Design review of the part built by this model. Coordinates are the model's own, in mm. Give positions to 0.01 mm unless a question says otherwise; leave off trailing zeros. Write each loop counter-clockwise with the first axis right and the second up, starting at its lowest first coordinate (ties: lowest second). Pieces come first, ordered by that corner, then holes. Notation, with made-up numbers: (76, -17.5) -> (133, -17.5) arc R9 ccw to (133, -3.5) -> close; hole circle Ø9 at (35.5, 29). An arc over 180 degrees is marked (long way). Put each result on its own line as item: value. Start each with the question number.
Autodesk Inventor part; units mm, degrees
ref_plane "YZ Plane" through (0, 0, 0) normal (1, 0, 0) x (0, 1, 0)
ref_plane "XZ Plane" through (0, 0, 0) normal (0, 1, 0) x (-1, 0, 0)
ref_plane "XY Plane" through (0, 0, 0) normal (0, 0, 1) x (1, 0, 0)
sketch "Sketch1" plane through (0, 0, 0) normal (0, 0, 1) x (1, 0, 0)
  circle A0 centre (46.9462, 34.742) radius 1.05
  circle A1 centre (53.415, 34.1058) radius 1.05
  circle A2 centre (-46.9442, -34.742) radius 1.05 construction
  circle A3 centre (-53.413, -34.1058) radius 1.05 construction
  arc A4 (72.8682, -20.1426) -> (68.7671, -31.41) centre (71.0414, -25.8577) ccw
  arc A5 (72.8682, -20.1426) -> (72.8688, 20.1405) centre (0.001, 0) ccw
  arc A6 (68.768, 31.408) -> (72.8688, 20.1405) centre (71.0421, 25.8557) ccw
  arc A7 (68.768, 31.408) -> (61.5859, 43.8482) centre (0.001, 0) ccw
  arc A8 (53.8786, 53.0336) -> (61.5859, 43.8482) centre (57.9147, 48.5939) ccw
  arc A9 (53.8786, 53.0336) -> (42.8749, 62.2671) centre (0.001, 0) ccw
  arc A10 (32.4909, 68.2625) -> (42.8749, 62.2671) centre (37.8019, 65.471) ccw
  arc A11 (32.4909, 68.2625) -> (18.9927, 73.1756) centre (0.001, 0) ccw
  arc A12 (7.1843, 75.258) -> (18.9927, 73.1756) centre (13.1299, 74.4513) ccw
  arc A13 (7.1843, 75.258) -> (-7.1802, 75.2582) centre (0.001, 0) ccw
  arc A14 (-18.9886, 73.1762) -> (-7.1802, 75.2582) centre (-13.1257, 74.4517) ccw
  arc A15 (-18.9886, 73.1762) -> (-32.4869, 68.2634) centre (0.001, 0) ccw
  arc A16 (-42.8711, 62.2683) -> (-32.4869, 68.2634) centre (-37.7981, 65.4721) ccw
  arc A17 (-42.8711, 62.2683) -> (-53.8751, 53.0351) centre (0.001, 0) ccw
  arc A18 (-61.5826, 43.8499) -> (-53.8751, 53.0351) centre (-57.9113, 48.5956) ccw
  arc A19 (-61.5826, 43.8499) -> (-68.7651, 31.41) centre (0.001, 0) ccw
  arc A20 (-72.8662, 20.1426) -> (-68.7651, 31.41) centre (-71.0394, 25.8577) ccw
  arc A21 (-72.8662, 20.1426) -> (-72.8668, -20.1405) centre (0.001, 0) ccw
  arc A22 (-68.766, -31.408) -> (-72.8668, -20.1405) centre (-71.0401, -25.8557) ccw
  arc A23 (-68.766, -31.408) -> (-61.5839, -43.8482) centre (0.001, 0) ccw
  arc A24 (-53.8766, -53.0336) -> (-61.5839, -43.8482) centre (-57.9127, -48.5939) ccw
  arc A25 (-53.8766, -53.0336) -> (-42.8729, -62.2671) centre (0.001, 0) ccw
  arc A26 (-32.4889, -68.2625) -> (-42.8729, -62.2671) centre (-37.7999, -65.471) ccw
  arc A27 (-32.4889, -68.2625) -> (-18.9907, -73.1756) centre (0.001, 0) ccw
  arc A28 (-7.1823, -75.258) -> (-18.9907, -73.1756) centre (-13.1279, -74.4513) ccw
  arc A29 (-7.1823, -75.258) -> (7.1822, -75.2582) centre (0.001, 0) ccw
  arc A30 (18.9906, -73.1762) -> (7.1822, -75.2582) centre (13.1277, -74.4517) ccw
  arc A31 (18.9906, -73.1762) -> (32.4889, -68.2634) centre (0.001, 0) ccw
  arc A32 (42.8731, -62.2683) -> (32.4889, -68.2634) centre (37.8001, -65.4721) ccw
  arc A33 (42.8731, -62.2683) -> (53.8771, -53.0351) centre (0.001, 0) ccw
  arc A34 (61.5846, -43.8499) -> (53.8771, -53.0351) centre (57.9133, -48.5956) ccw
  arc A35 (61.5846, -43.8499) -> (68.7671, -31.41) centre (0.001, 0) ccw
  circle A36 centre (0.001, 0) radius 44.3
  circle A37 centre (-69.9492, -11.499) radius 1.3
  circle A38 centre (-46.9488, 11.5007) radius 1.3
  circle A39 centre (69.9508, -11.501) radius 1.3
  circle A40 centre (46.9512, 11.4993) radius 1.3
  circle A41 centre (69.9512, 11.499) radius 1.3
  circle A42 centre (46.9508, -11.5007) radius 1.3
  circle A43 centre (-69.9488, 11.501) radius 1.3
  circle A44 centre (-46.9492, -11.4993) radius 1.3
  circle A45 centre (-58.449, 0.0008) radius 11.5
  circle A46 centre (58.451, -0.0008) radius 11.5
  circle A47 centre (60.2759, -34.8009) radius 1.55
  circle A48 centre (44.7383, -53.3173) radius 1.55
  circle A49 centre (16.1779, -44.4477) radius 1.55
  circle A50 centre (0, -69.6) radius 1.55
  circle A51 centre (-23.8045, -65.4023) radius 1.55
  circle A52 centre (-30.4034, -36.2335) radius 1.55
  circle A53 centre (-60.2749, -34.7991) radius 1.55
  circle A54 centre (60.2769, 34.7991) radius 1.55
  circle A55 centre (44.7398, 53.3161) radius 1.55
  circle A56 centre (23.8065, 65.4023) radius 1.55
  circle A57 centre (-40.9617, 23.6506) radius 1.55
  circle A58 centre (-30.4023, 36.2343) radius 1.55
  circle A59 centre (-16.1759, 44.4477) radius 1.55
  circle A60 centre (0.0017, 47.3) radius 1.55
  circle A61 centre (0.002, 69.6) radius 1.55
  circle A62 centre (-23.8027, 65.4029) radius 1.55
  circle A63 centre (-44.7363, 53.3173) radius 1.55
  circle A64 centre (-60.2739, 34.8009) radius 1.55
  circle A65 centre (16.1792, 44.4472) radius 1.55
  circle A66 centre (30.4054, 36.2335) radius 1.55
  circle A67 centre (40.9643, 23.6494) radius 1.55
  circle A68 centre (-40.9623, -23.6494) radius 1.55
  circle A69 centre (-44.7378, -53.3161) radius 1.55
  circle A70 centre (-16.1772, -44.4472) radius 1.55
  circle A71 centre (0.0003, -47.3) radius 1.55
  circle A72 centre (23.8047, -65.4029) radius 1.55
  circle A73 centre (30.4043, -36.2343) radius 1.55
  circle A74 centre (40.9637, -23.6506) radius 1.55
  line L0 (58.451, 0) -> (0.001, 0) construction
  line L1 (71.0414, -19.8577) -> (39.601, -19.8577)
  line L2 (0.001, 0) -> (0.001, -87.4041) construction
  line L3 (71.0414, -25.8577) -> (71.0414, -19.8577) construction
  line L4 (39.601, -19.8577) -> (-39.599, -19.8577) construction
  line L5 (-39.599, -19.8577) -> (-71.0397, -19.8557)
  point P0 (0, 0)
extrude "Extrusion1" add sketch "Sketch1" along normal blind 1.75 contours A4 A35 A34 A33 A32 A31 A30 A29 A28 A27 A26 A25 A24 A23 A22 L5 A36 L1
sketch "Sketch2" plane through (0, 0, 1.75) normal (0, 0, 1) x (1, 0, 0)
  circle A0 centre (-30.4034, -36.2335) radius 1.55
  circle A1 centre (-44.7378, -53.3161) radius 1.55
  circle A2 centre (-23.8045, -65.4023) radius 1.55
  circle A3 centre (-16.1772, -44.4472) radius 1.55
  circle A4 centre (16.1779, -44.4477) radius 1.55
  circle A5 centre (23.8047, -65.4029) radius 1.55
  circle A6 centre (44.7383, -53.3173) radius 1.55
  circle A7 centre (30.4043, -36.2343) radius 1.55
  circle A8 centre (0.0003, -47.3) radius 1.55
  point P0 (0, 0)
extrude "Extrusion2" add sketch "Sketch2" against normal up to surface (1.75 mm away)
sketch "Sketch3" plane through (0, 0, 1.75) normal (0, 0, 1) x (1, 0, 0)
  line L0 (-60.9088, -23.5183) -> (-47.1121, -23.5183) construction
  line L1 (-60.9088, -25.0183) -> (-47.1121, -25.0183)
  line L2 (-47.1121, -22.0183) -> (-60.9088, -22.0183)
  arc A0 (-60.9088, -22.0183) -> (-60.9088, -25.0183) centre (-60.9088, -23.5183) ccw
  arc A1 (-47.1121, -25.0183) -> (-47.1121, -22.0183) centre (-47.1121, -23.5183) ccw
  line L3 (-60.9088, -23.5183) -> (-65.5141, -23.5183) construction
  arc A2 (-68.766, -31.408) -> (-71.0397, -19.8557) centre (-71.0401, -25.8557) ccw
  line L4 (-47.1121, -23.5183) -> (-42.5068, -23.5183) construction
  circle A3 centre (-40.9623, -23.6494) radius 1.55
  point P0 (0, 0)
  point P1 (-54.0105, -23.5183)
  point P2 (-71.0401, -19.8557)
  dimension "d4" = 3
extrude "Extrusion3" cut sketch "Sketch3" against normal up to surface (1.75 mm away) contours A0 L2 A1 L1
mirror "Mirror1" about plane through (0, 0, 0) normal (1, 0, 0) of "Extrusion3"
sketch "Sketch4" plane through (0, 0, 1.75) normal (0, 0, 1) x (1, 0, 0)
  line L0 (13.6094, 45.369) -> (8.7511, 46.5508) construction
  line L1 (13.8458, 46.3407) -> (8.9875, 47.5225)
  line L2 (8.5148, 45.5792) -> (13.3731, 44.3973)
  arc A0 (13.3731, 44.3973) -> (13.8458, 46.3407) centre (13.6094, 45.369) ccw
  arc A1 (8.9875, 47.5225) -> (8.5148, 45.5792) centre (8.7511, 46.5508) ccw
  circle A2 centre (0, 0) radius 47.3002 construction
  arc A3 (-39.599, -19.8577) -> (39.601, -19.8577) centre (0.001, 0) ccw
  point P0 (11.1803, 45.9599)
  point P1 (-39.6, -19.8557)
  dimension "d7" = 2
  dimension "d8" = 5
  dimension "d9" = 2
extrude "Extrusion4" cut sketch "Sketch4" against normal up to surface (1.75 mm away)
equation "\"d0\" = board_height"
equation "\"d2\" = board_height"
equation "\"d5\" = board_height"
equation "\"d10\" = board_height"
equation "\"board_height\" = 1.75"
properties part number "Board_Shape"
Q1. Mouldability with a two-part tool opening along Y and no side actions: class faces 1 (the face through (-42.51, -23.72, 0.86)), 2 (the face through (-1, -47, 0)), 3 (the face through (65.522, -37.714, 0.863)) as +Y half, -Y half, draft (parallel to the pull), parting line (faces both ways), or undercut.
Q2. To check wall thickness, follow probe 1 along X at (y, z) = (-35, 0.4); probe 2 along Y at (x, z) = (0, 0.6); probe 3 along X at (y, z) = (-31, 1.7). State the ranges of each line that lie inside material, in increasing order. Write a range as from..to.
Q3. Take a section at B-B on z = 1.05. State how many separate pieces and enclosed holes the cut face has, then the cut area to 3 significant figures.
Q4. Take a section at D-D on x = -16. Give the boundary of the cut face in (y, z), then the cut area to 3 significant figures.
Q5. For pin 1 (1 mm diameter, centred on x = 22, z = 1, fed in from +Y); pin 2 (3.5 mm diameter, centred on x = 0, y = -69.6, fed in from +Z); pin 3 (0.9 mm diameter, centred on x = -53, z = 0.5, fed in from -Y); pin 4 (1 mm diameter, centred on x = 3, z = 1.5, fed in from +Y), all flat-tipped, find the tip position at first contact; note any pin that passes through.
Q6. Take a section at A-A on x = 0. Give the boundary of the cut face in (y, z), then the cut area to 4 significant figures.
Q7. Take a section at C-C on y = -56. Give the boundary of the cut face in (x, z), then the cut area to 3 significant figures.
Result:
1. face 1: undercut
1. face 2: draft
1. face 3: -Y half
2. probe 1: x = -67.01..-61.81, -58.74..-27.16, 27.16..58.74, 61.81..67.01
2. probe 2: y = -75.6..-71.15, -68.05..-44.3
2. probe 3: x = -67.95..-31.65, 31.65..67.95
3. separate pieces: 1
3. enclosed holes: 7
3. area: 4,050 mm^2
4. outline: (-69.18, 0) -> (-41.31, 0) -> (-41.31, 1.75) -> (-69.18, 1.75) -> close
4. area: 48.8 mm^2
5. pin 1: stops at y = -38.16
5. pin 2: stops at z = 1.75
5. pin 3: stops at y = -54.35
5. pin 4: stops at y = -44.16
6. outline: (-75.6, 0) -> (-71.15, 0) -> (-71.15, 1.75) -> (-75.6, 1.75) -> close; (-68.05, 0) -> (-44.3, 0) -> (-44.3, 1.75) -> (-68.05, 1.75) -> close
6. area: 49.35 mm^2
7. outline: (-50.79, 0) -> (50.79, 0) -> (50.79, 1.75) -> (-50.79, 1.75) -> close
7. area: 178 mm^2
